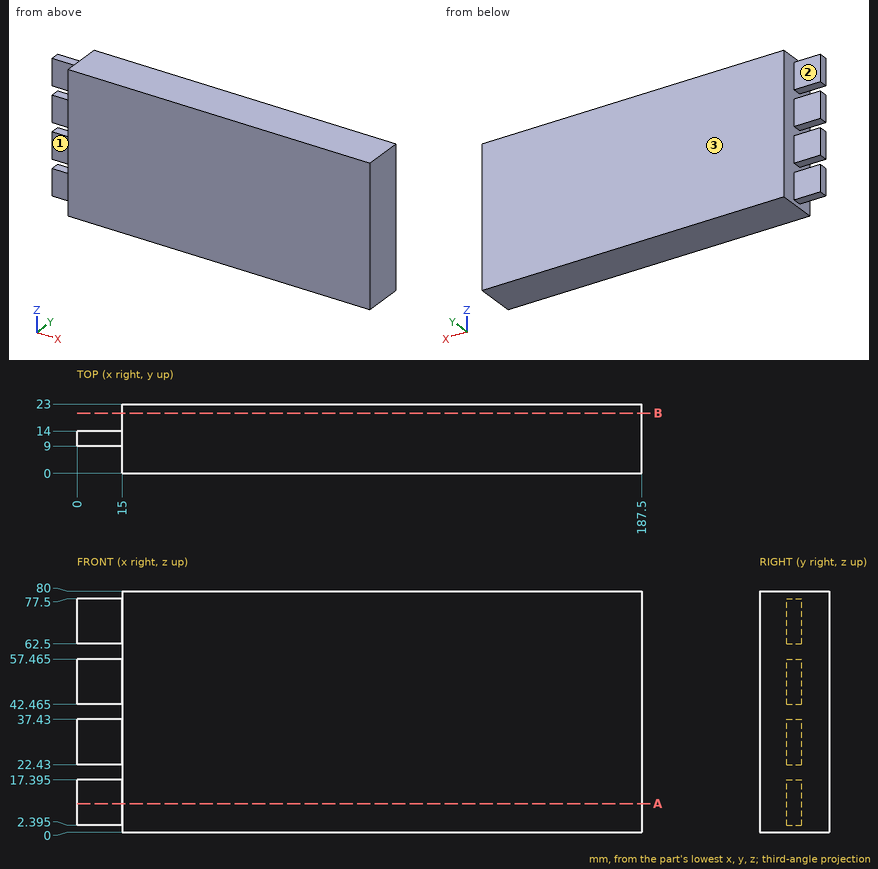
Input: dimensioned drawing with shaded views. Units: mm. Origin: part minimum x, y, z. A direction names the side the tool comes from. Coordinates: 2 decimals unless noted, no trailing zeros. Order: outer loops, then holes, each group sorted by start corner. A loop starts at its lowest first (then second) coordinate and runs counter-clockwise, first axis right, second up. Notation, with made-up numbers: (12, -26) -> (48, -26) arc R19 ccw to (48, -16) -> close; hole circle Ø3 at (75.5, -4). An arc over 180 degrees is marked (long way). Use CSV: the item, a comma, the result in double quotes.
1) Line query: line 1 (X direction, y = 6.5, z = 41); line 2 (Y direction, x = 11.5, z = 5). Output: solid intervals per line, ascending.
Findings:
line 1,"x = 15 to 187.5"
line 2,"y = 9 to 14"
2) Section B-B on y = 20. Output: boundary loops of the cut face in (x, z).
Findings:
outline,"(15, 0) -> (187.5, 0) -> (187.5, 80) -> (15, 80) -> close"
3) Access query for the marked faces 1, 2 and 3. Directions: +Z, -Z, +X, -X, +Y, -Y. A direction counts if a zero-diameter tool reaches every point of the face in a straight line with its end or side. Return the directions, or none.
Findings:
face 1,"+Z, -Z, -X, -Y"
face 2,"+Z, -Z, -X, +Y"
face 3,"+Z, -Z, +X, -X, +Y"
4) Section A-A on z = 9.5. Output: boundary loops of the cut face in (x, y).
Findings:
outline,"(0, 9) -> (15, 9) -> (15, 0) -> (187.5, 0) -> (187.5, 23) -> (15, 23) -> (15, 14) -> (0, 14) -> close"
5) Pin query (flat end, axial travel): pin 1 Ø12 at (x, z) = (6.5, 72) entering from -Y; pin 2 Ø2.5 at (x, y) = (10.5, 11) entering from +Z; pin 3 Ø12 at (y, z) = (2.5, 61) entering from -X. Return the tip coordinate at first contact, or that it passes through.
Findings:
pin 1,"stops at y = 9"
pin 2,"stops at z = 77.5"
pin 3,"stops at x = 15"
